Study the drawing (mm; zero at the part's minimum x, y, z) and answer. Coordinates: 2 decimals unless noted, no trailing zeros. Order: outer loops, then holes, each group sorted by start corner. A loop starts at its lowest first (then second) coordinate and runs counter-clockwise, first axis right, second up.
1. Flat-ended cylindrical pins translate along their axes: pin 1 Ø2 at (x, y) = (1.5, 23) entering from -Z; pin 2 Ø4 at (y, z) = (48.5, 73) entering from +X; pin 3 Ø1.2 at (x, y) = (2, 24) entering from +Z; pin 4 Ø2 at (x, z) = (1.5, 68.5) entering from -Y. Find the tip coordinate at first contact, or state that the pin passes through.
2. The part is cut by section A-A, the plane x = 1.9. Give the vertices of the cut face in (y, z), then the cut area to 3 significant figures.
3. The part is cut by section B-B, the plane y = 36. Give the vertices of the cut face in (x, z), then the cut area to 3 significant figures.
4. The part is cut by section D-D, the plane y = 48.5. Give the vertices of the cut face in (x, z), then the cut area to 3 significant figures.
5. The part is cut by section C-C, the plane z = 7. Give the vertices of the cut face in (x, y).
6. Find the intervals of material crossed by probe 1 along Y at (x, z) = (1.1, 40); probe 2 along Y at (x, z) = (0.45, 13); probe 3 along Z at (x, y) = (1.2, 60.5), in increasing order.
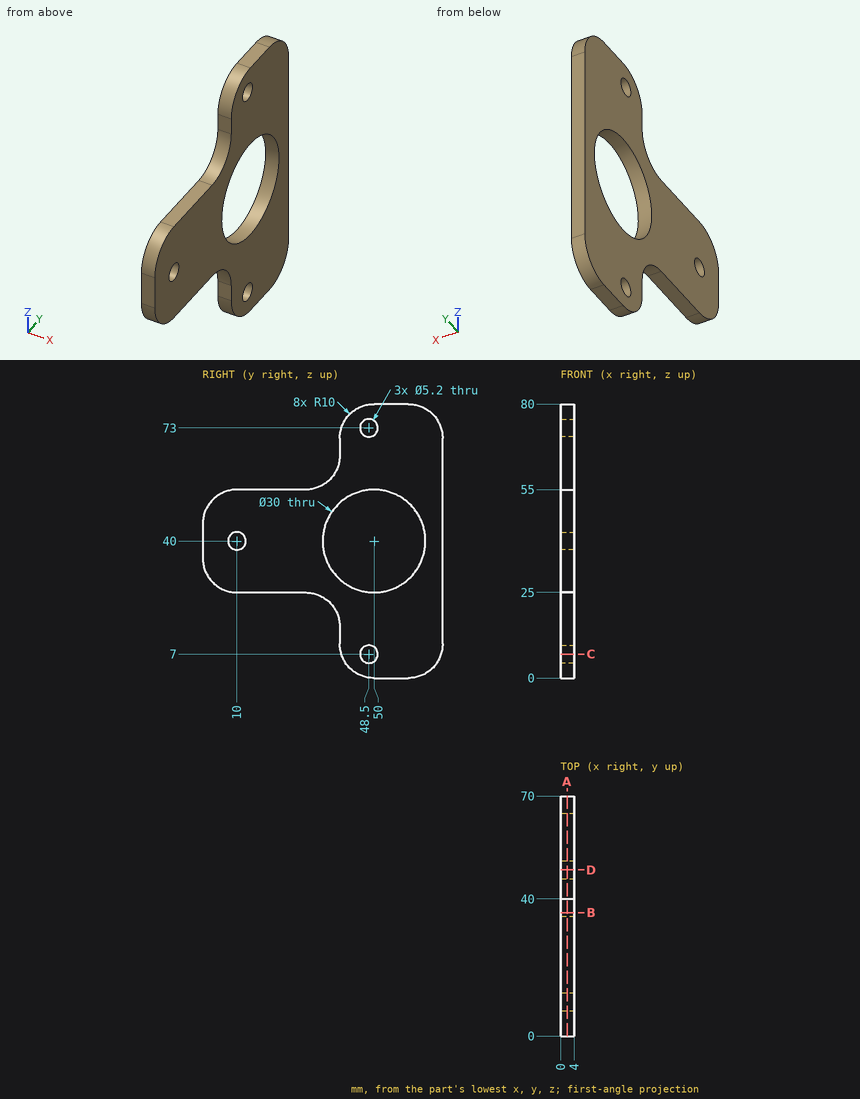
Geometry says:
1. pin 1: stops at z = 25
1. pin 2: passes through
1. pin 3: stops at z = 55
1. pin 4: stops at y = 40
2. outline: (0, 35) arc R10 ccw to (10, 25) - (30, 25) arc R10 cw to (40, 15) - (40, 10) arc R10 ccw to (50, 0) - (60, 0) arc R10 ccw to (70, 10) - (70, 70) arc R10 ccw to (60, 80) - (50, 80) arc R10 ccw to (40, 70) - (40, 65) arc R10 cw to (30, 55) - (10, 55) arc R10 ccw to (0, 45) - close; hole circle Ø5.2 at (10, 40); hole circle Ø30 at (50, 40); hole circle Ø5.2 at (48.5, 7); hole circle Ø5.2 at (48.5, 73)
2. area: 2,740 mm2
3. outline: (0, 23) - (4, 23) - (4, 34.61) - (0, 34.61) - close; (0, 45.39) - (4, 45.39) - (4, 57) - (0, 57) - close
3. area: 92.9 mm2
4. outline: (0, 0.11) - (4, 0.11) - (4, 4.4) - (0, 4.4) - close; (0, 9.6) - (4, 9.6) - (4, 25.08) - (0, 25.08) - close; (0, 54.92) - (4, 54.92) - (4, 70.4) - (0, 70.4) - close; (0, 75.6) - (4, 75.6) - (4, 79.89) - (0, 79.89) - close
4. area: 158 mm2
5. outline: (0, 40.46) - (4, 40.46) - (4, 45.9) - (0, 45.9) - close; (0, 51.1) - (4, 51.1) - (4, 69.54) - (0, 69.54) - close
6. probe 1: y = 0 to 7.4, 12.6 to 35, 65 to 70
6. probe 2: y = 40 to 70
6. probe 3: z = 0.01 to 29.29, 50.71 to 79.99
